Print and shaded views of the part. All mm, measured from the part's lowest x, y and z. A direction names the side the tool comes from. Coordinates: 2 decimals unless noted, no trailing zeros. Loops run counter-clockwise (first coordinate to the right, second up) from the corner with the lowest first, then second, coordinate; pieces in that order, holes last.
1) Saw through at B-B, the plane x = 25. Write the cut outline in (y, z), and give its area (3 significant figures).
2) Pin check, flat tips, straight feed: pin 1 Ø1 at (x, z) = (22.5, 4) entering from +Y; pin 2 Ø5.5 at (x, z) = (21, 6) entering from -Y. Stop position of each tip, or through.
3) Saw through at A-A, the plane y = 12.25. Write the cut outline in (x, z), and give its area (3 significant figures).
4) Two-plate mould, pull along Z, no slides. Class the marked faces 4, 5, 6 and 7: +Z half, -Z half, draft (parallel to the pull), parting line (faces both ways), or undercut.
5) Wall check: line 1 along Z through (x, y) = (11.25, 10.75); line 2 along X through (y, z) = (18, 13.75); line 3 along Y through (x, z) = (7, 7). Give the ranges that are in metal, low to high.
6) Which spindle directions (+Z, -Z, +X, -X, +Y, -Y) get a long thin tool onto all of the face, cutting with end or side? Do the marked faces 1, 2 and 3. Say none if no direction does.
7) Saw through at C-C, the plane z = 14.9. Write the cut outline in (x, y), and give its area (3 significant figures).
8) Saw through at D-D, the plane x = 19.45. Write the cut outline in (y, z).
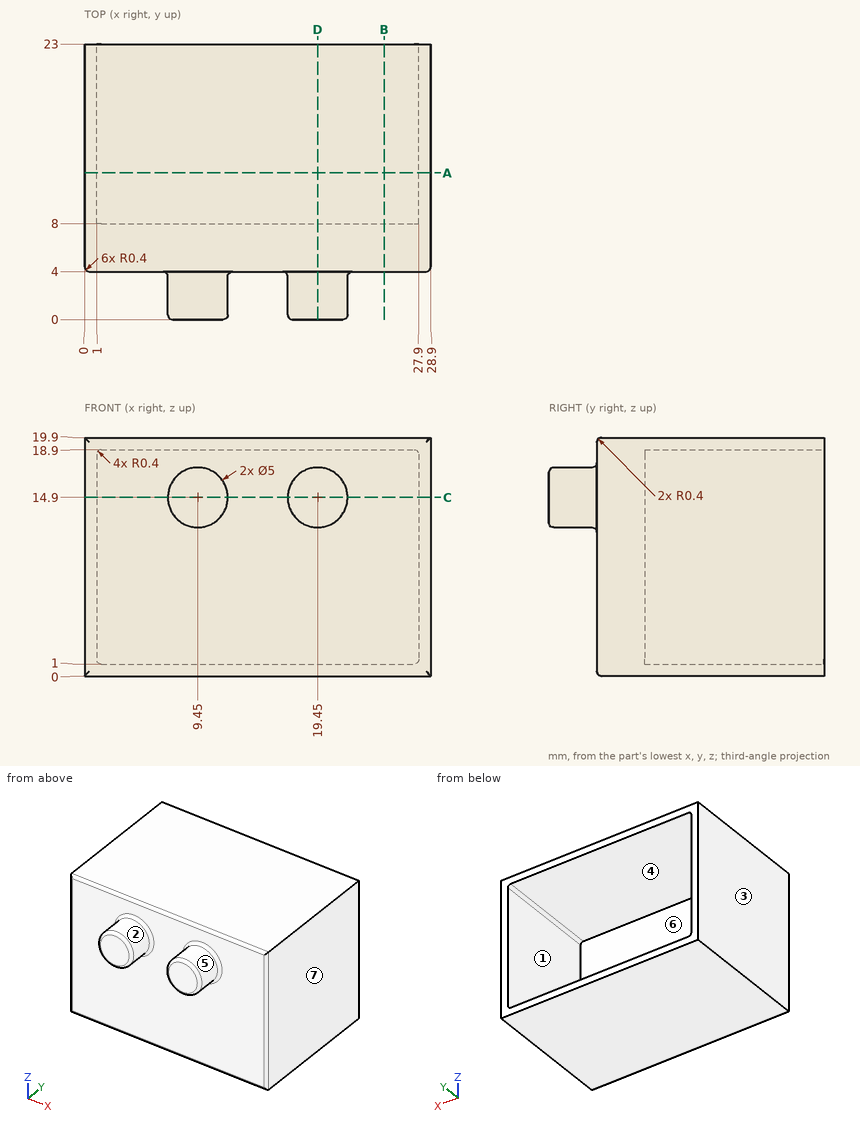
Data:
1. outline: (4, 0.4) arc R0.4 ccw to (4.4, 0) - (23, 0) - (23, 1) - (8, 1) - (8, 18.9) - (23, 18.9) - (23, 19.9) - (4.4, 19.9) arc R0.4 ccw to (4, 19.5) - close
1. area: 110 mm2
2. pin 1: stops at y = 8
2. pin 2: stops at y = 4
3. outline: (0, 0) - (28.9, 0) - (28.9, 19.9) - (0, 19.9) - close; hole (1, 1.4) arc R0.4 ccw to (1.4, 1) - (27.5, 1) arc R0.4 ccw to (27.9, 1.4) - (27.9, 18.5) arc R0.4 ccw to (27.5, 18.9) - (1.4, 18.9) arc R0.4 ccw to (1, 18.5) - close
3. area: 93.7 mm2
4. face 4: undercut
4. face 5: parting line
4. face 6: undercut
4. face 7: draft
5. line 1: z = 0 to 1, 18.9 to 19.9
5. line 2: x = 0 to 1, 27.9 to 28.9
5. line 3: y = 4 to 8
6. face 1: +Y
6. face 2: -Y
6. face 3: +Z, -Z, -X, +Y, -Y
7. outline: (0, 4.4) arc R0.4 ccw to (0.4, 4) - (6.55, 4) arc R0.4 cw to (6.95, 3.6) - (6.95, 0.4) arc R0.4 ccw to (7.35, 0) - (11.55, 0) arc R0.4 ccw to (11.95, 0.4) - (11.95, 3.6) arc R0.4 cw to (12.35, 4) - (16.55, 4) arc R0.4 cw to (16.95, 3.6) - (16.95, 0.4) arc R0.4 ccw to (17.35, 0) - (21.55, 0) arc R0.4 ccw to (21.95, 0.4) - (21.95, 3.6) arc R0.4 cw to (22.35, 4) - (28.5, 4) arc R0.4 ccw to (28.9, 4.4) - (28.9, 23) - (27.9, 23) - (27.9, 8) - (1, 8) - (1, 23) - (0, 23) - close
7. area: 186 mm2
8. outline: (0, 12.8) arc R0.4 ccw to (0.4, 12.4) - (3.6, 12.4) arc R0.4 cw to (4, 12) - (4, 0.4) arc R0.4 ccw to (4.4, 0) - (23, 0) - (23, 1) - (8, 1) - (8, 18.9) - (23, 18.9) - (23, 19.9) - (4.4, 19.9) arc R0.4 ccw to (4, 19.5) - (4, 17.8) arc R0.4 cw to (3.6, 17.4) - (0.4, 17.4) arc R0.4 ccw to (0, 17) - close
